Design review of the part built by this model. Coordinates are the model's own, in mm. Face numbers are marked on the shaded views. A direction names the side the tool comes from. Coordinates: 2 decimals unless noted, no trailing zeros. Write each loop counter-clockwise with the first axis right and the second up, starting at its lowest first coordinate (ties: lowest second). Pieces come first, ordered by that corner, then holes. Notation, with made-up numbers: (50, 26) -> (79, 26) arc R22 cw to (79, 37) -> close; hole circle Ø10 at (42.5, -5.75). An arc over 180 degrees is marked (long way). One line per question, with ' | ' between items. Start each with the question number.
Q1. Draft analysis for pull direction Y (two halves, no side actions). For the marked faces 3, 4, 5 and 6, state which applies: pulls with the +Y half, pulls with the -Y half, needs draft (parallel to the pull), parting line crosses it, or undercut.
Q2. For P1, Ø2, axis at x = 24, y = -17.5, coming from the +Z side; P2, Ø1.5, axis at x = -12, y = -14, coming from the +Z side; P3, Ø5.5, axis at x = -25, y = -17.1, coming from the -Z side; P4, Ø6, axis at x = -13, z = -6, coming from the +Y side, all flat-tipped, find the tip position at first contact; note any pin that passes through.
Q3. Add section D-D on z = 8. State the section outline as (x, y) points, and give its area (3 significant figures).
Q4. Add section C-C on x = 24.9. State the section outline as (y, z) points.
Q5. Add section B-B on z = -10.5. State the section outline as (x, y) points, and give its area (3 significant figures).
Q6. Add section A-A on z = 22.5. State the section outline as (x, y) points, and give its area (3 significant figures).
Q7. Wall thickness on probe 1 along X at (y, z) = (-7.2, 22.25); probe 2 along Y at (x, z) = (11, -10); probe 3 along Y at (x, z) = (24.9, 20.75): over which ranges is each line inside the solid? List them lowest first.
Q8. For the marked faces 1 and 2, list the 3-axis set-ups (+Z, -Z, +X, -X, +Y, -Y) from which the entire face can be reached by the end or side of a thin tool; tool diameter is ignored.
from build123d import *

# Parameters (mm, degrees)
PAD_DEPTH       = 24
SKETCH003_W     = 42
SKETCH003_H     = 1.8
PAD002_DEPTH    = 30
SKETCH001_R     = 10
POCKET_DEPTH    = 5
SKETCH004_R     = 7.75
PAD003_DEPTH    = 25
SKETCH005_R     = 2.000122
SKETCH005_R_2   = 2.001214
SKETCH005_R_3   = 2.1
SKETCH005_R_4   = 2.10238
POCKET001_DEPTH = 10


with BuildPart() as part:
    # Sketch → Pad (new body)
    with BuildSketch(Plane.XZ):
        Polygon((-21.000973, 28), (-29, 28), (-29, -2), (-29, -12), (29, -12), (29, 28), (21, 28), (21, -2), (-21.000973, -2), align=None)
    extrude(amount=PAD_DEPTH)

    # Sketch003 → Pad002 (join)
    with BuildSketch(Plane(origin=(0, 0, -2), x_dir=(-1, 0, 0), z_dir=(0, 0, 1))):
        with Locations((0, 0.9)):
            Rectangle(SKETCH003_W, SKETCH003_H)
        with Locations((0, 23.1)):
            Rectangle(SKETCH003_W, SKETCH003_H)
    extrude(amount=PAD002_DEPTH)

    # Sketch001 (on Face5 of Pad) → Pocket (cut)
    with BuildSketch(Plane(origin=(0, 0, -12), x_dir=(1, 0, 0), z_dir=(0, 0, -1))):
        with Locations((11, 12)):
            Circle(SKETCH001_R)
    extrude(amount=-POCKET_DEPTH, mode=Mode.SUBTRACT)

    # Sketch004 (on Face21 of Pocket) → Pad003 (join)
    with BuildSketch(Plane(origin=(0, 0, -7), x_dir=(1, 0, 0), z_dir=(0, 0, -1))):
        with Locations((11, 12)):
            Circle(SKETCH004_R)
    extrude(amount=PAD003_DEPTH)

    # Sketch005 (on Face15 of Pad003) → Pocket001 (cut)
    with BuildSketch(Plane(origin=(0, 0, 28), x_dir=(-1, 0, 0), z_dir=(0, 0, 1))):
        with Locations((-24.9, 17.2)):
            Circle(SKETCH005_R)
        with Locations((-24.9, 7.2)):
            Circle(SKETCH005_R_2)
        with Locations((24.9, 7.2)):
            Circle(SKETCH005_R_3)
        with Locations((25, 17.1)):
            Circle(SKETCH005_R_4)
    extrude(amount=-POCKET001_DEPTH, mode=Mode.SUBTRACT)


solid = part.part
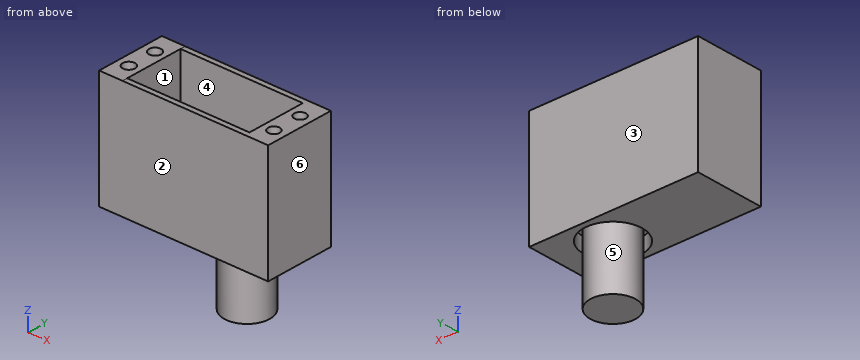
Output values:
1) face 3: pulls with the +Y half | face 4: undercut | face 5: undercut | face 6: needs draft
2) P1: stops at z = 18 | P2: stops at z = -2 | P3: stops at z = -12 | P4: stops at y = 0
3) outline: (-29, -24) -> (-21, -24) -> (-21, 0) -> (-29, 0) -> close; (-21, -24) -> (29, -24) -> (29, 0) -> (-21, 0) -> (-21, -1.8) -> (21, -1.8) -> (21, -22.2) -> (-21, -22.2) -> close | area: 535 mm2
4) outline: (-24, -12) -> (0, -12) -> (0, 28) -> (-5.2, 28) -> (-5.2, 18) -> (-9.2, 18) -> (-9.2, 28) -> (-15.2, 28) -> (-15.2, 18) -> (-19.2, 18) -> (-19.2, 28) -> (-24, 28) -> close
5) outline: (-29, -24) -> (29, -24) -> (29, 0) -> (-29, 0) -> close; circle Ø15.5 at (11, -12); hole circle Ø20 at (11, -12) | area: 1,270 mm2
6) outline: (-29, -24) -> (-21, -24) -> (-21, 0) -> (-29, 0) -> close; (-21, -24) -> (29, -24) -> (29, 0) -> (-21, 0) -> (-21, -1.8) -> (21, -1.8) -> (21, -22.2) -> (-21, -22.2) -> close; hole circle Ø4.2 at (-25, -17.1); hole circle Ø4.2 at (-24.9, -7.2); hole circle Ø4 at (24.9, -17.2); hole circle Ø4 at (24.9, -7.2) | area: 482 mm2
7) probe 1: x = -29 to -27, -22.8 to -21, 21 to 22.9, 26.9 to 29 | probe 2: y = -24 to -22, -19.75 to -4.25, -2 to 0 | probe 3: y = -24 to -19.2, -15.2 to -9.2, -5.2 to 0
8) face 1: none | face 2: +Z, -Z, +X, -X, -Y
